```python
from build123d import *

# Parameters (mm, degrees)
F0_R     = 63.5
F1_DEPTH = 7.62
F2_R     = 25.4
F3_DEPTH = 10.16
F5_DEPTH = 25.4


with BuildPart() as f1:
    # F0 (on Top) → F1 (new body)
    with BuildSketch(Plane.XY):
        with Locations((-7.679907, 7.63871)):
            Circle(F0_R)
    extrude(amount=F1_DEPTH)

    # F2 (on face) → F3 (cut)
    with BuildSketch(Plane.XY.offset(7.62)):
        with Locations((-7.679907, 7.63871)):
            Circle(F2_R)
    extrude(amount=-F3_DEPTH, mode=Mode.SUBTRACT)

    # F4 (on face) → F5 (cut)
    with BuildSketch(Plane.XY.offset(7.62)):
        Polygon((-70.018905, -10.474761), (-75.894549, -20.027222), (-70.559698, -29.89191), (-59.349201, -30.204137), (-53.473556, -20.651676), (-58.808408, -10.786988), align=None)
        Polygon((-72.942136, 3.63904), (-60.994428, 7.849691), (-58.667104, 20.302035), (-68.287489, 28.543728), (-80.235197, 24.333077), (-82.562521, 11.880733), align=None)
        Polygon((-63.660068, 38.412835), (-51.911708, 37.186518), (-44.975507, 46.747738), (-49.787665, 57.535274), (-61.536025, 58.761591), (-68.472226, 49.200372), align=None)
        Polygon((-23.294299, 79.663551), (-37.981644, 76.049112), (-39.082748, 60.963693), (-25.075922, 55.254831), (-15.318124, 66.811979), align=None)
        Polygon((-47.082333, -58.607126), (-33.286273, -64.939879), (-20.903919, -56.158517), (-22.317623, -41.044403), (-36.113683, -34.71165), (-48.496038, -43.493011), align=None)
        Polygon((5.356202, -68.9087), (20.162689, -64.180396), (23.471101, -48.993451), (11.973027, -38.53481), (-2.83346, -43.263113), (-6.141872, -58.450058), align=None)
        Polygon((34.981984, -41.765964), (48.281185, -43.091442), (56.078684, -32.236736), (50.576981, -20.056551), (37.27778, -18.731073), (29.480282, -29.585779), align=None)
        Polygon((52.745689, -11.753145), (69.391161, -5.659039), (72.436247, 11.803416), (58.83586, 23.171765), (42.190388, 17.077659), (39.145302, -0.384796), align=None)
        Polygon((48.057828, 35.814065), (55.786416, 49.200372), (48.057828, 62.586678), (32.600653, 62.586678), (24.872065, 49.200372), (32.600653, 35.814065), align=None)
        Polygon((20.397003, 66.884476), (16.08287, 79.105869), (3.341766, 81.480417), (-5.085204, 71.633571), (-0.771071, 59.412177), (11.970033, 57.03763), align=None)
    extrude(amount=-F5_DEPTH, mode=Mode.SUBTRACT)


solid = f1.part
```
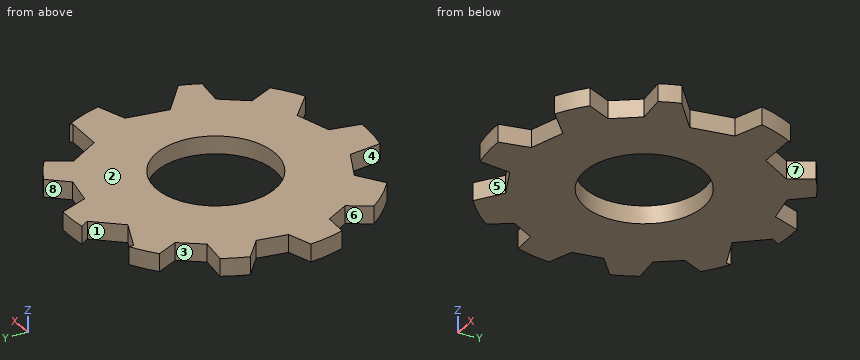
Work out the finished part from the listing and answer in its coordinate system (mm). Face numbers are marked on the shaded views. A direction names the side the tool comes from. Give positions to 0.01 mm unless a question says otherwise; leave off trailing zeros. Loops run counter-clockwise (first coordinate to the right, second up) from the corner with the lowest first, then second, coordinate; pieces in that order, holes last. Notation, with made-up numbers: (-20, 35) -> (17, 35) arc R8 ccw to (17, 48) -> close; hole circle Ø7 at (2, -23). An arc over 180 degrees is marked (long way). One line per question, with ' | ' between items. Start each with the question number.
1) Section B-B, the plane y = -4 is taken. Determine the outline of the cut face in (x, z), then the cut area to 3 significant figures.
2) Section D-D, the plane x = 21 is taken. Determine the outline of the cut face in (y, z).
3) For the marked faces 5, 6, 7 and 8, determine the directions among +Z, -Z, +X, -X, +Y, -Y from which every point of the face is accessible in a straight line to the end or side of a thin tool.
4) Section C-C, the plane y = -32 is taken. Determine the outline of the cut face in (x, z).
5) Section A-A, the plane x = 5 is taken. Determine the outline of the cut face in (y, z), then the cut area to 3 significant figures.
6) Straight lines are drawn through the part: L1, parallel to X at y = -6.5, z = 1.25; L2, parallel to Y at x = 28, z = 1.5; L3, parallel to X at y = -5, z = 1. For each, find the intervals that lie inside material, in ascending order.
7) Determine the mould class of the marked faces 1, 2, 3 and 4 for opening direction Y: +Y half, -Y half, draft (parallel to the pull), parting line (faces both ways), or undercut.
8) Each of these flat-tipped pins is pushed along its axis until it touches: pin 1 (1 mm diameter, centred on y = -20.5, z = 5.5, fed in from +X); pin 2 (4 mm diameter, centred on x = 29.5, z = 3.5, fed in from +Y); pin 3 (4 mm diameter, centred on y = -20.5, z = 1.5, fed in from -X). Where does it stop, or does it pass through?
Resolved:
1) outline: (-70.1, 0) -> (-30.26, 0) -> (-30.26, 7.62) -> (-70.1, 7.62) -> close; (14.9, 0) -> (43.47, 0) -> (43.47, 7.62) -> (14.9, 7.62) -> close | area: 521 mm2
2) outline: (-46.75, 0) -> (64.29, 0) -> (64.29, 7.62) -> (-46.75, 7.62) -> close
3) face 5: +Z, -Z, -Y | face 6: +Z, -Z, -X | face 7: +Z, -Z, +X | face 8: +Z, -Z, +Y
4) outline: (-57.29, 0) -> (30.57, 0) -> (30.57, 7.62) -> (-57.29, 7.62) -> close
5) outline: (-40.76, 0) -> (-14.37, 0) -> (-14.37, 7.62) -> (-40.76, 7.62) -> close; (29.65, 0) -> (58.34, 0) -> (58.34, 7.62) -> (29.65, 7.62) -> close | area: 420 mm2
6) L1: -69.59 to -28.78, 13.42 to 46.46 | L2: -44.89 to 43.78, 54.62 to 60.17 | L3: -69.91 to -29.71, 14.35 to 44.67
7) face 1: undercut | face 2: draft | face 3: undercut | face 4: -Y half
8) pin 1: x = 36.37 | pin 2: y = 60.5 | pin 3: x = -54.64
